Input: part model. Units: mm. Frame: model coordinates. Coordinates: 2 decimals unless noted, no trailing zeros. Write each loop counter-clockwise with the first axis right and the second up, starting at its lowest first coordinate (ties: lowest second). Pieces come first, ordered by that corner, then holes.
1) Section query B-B (z = 2.5). Output: boundary loops of the cut face in (x, y).
2) Section query D-D (x = -137). Output: boundary loops of the cut face in (y, z).
3) Section query C-C (y = 104). Output: boundary loops of the cut face in (x, z), then the cut area to 3 significant figures.
4) Section query A-A (x = -72.5). Output: boundary loops of the cut face in (y, z).
5) Line query: L1, parallel to Y at x = -47.5, z = 1.2; L2, parallel to X at y = 121, z = 0.85; L3, parallel to Y at x = -73, z = 1.75. Output: solid intervals per line, ascending.
from build123d import *

# Parameters (mm, degrees)
SKETCH_1_R      = 2.5
EXTRUDE_1_DEPTH = 4


with BuildPart() as part:
    # 草图1 → 凸台-拉伸1 (new body)
    with BuildSketch(Plane.XY):
        with BuildLine():
            Line((-11.50990482, 0), (-108.49009518, 0))
            ThreePointArc((-108.49009518, 0), (-117.621516615, 3.099699896), (-122.978982575, 11.117714323))
            Line((-122.978982575, 11.117714323), (-154.940506802, 130.399746626))
            ThreePointArc((-154.940506802, 130.399746626), (-152.351919512, 143.413453738), (-140.451619407, 149.282032303))
            Line((-140.451619407, 149.282032303), (20.451619407, 149.282032303))
            ThreePointArc((20.451619407, 149.282032303), (32.351919512, 143.413453738), (34.940506802, 130.399746626))
            Line((34.940506802, 130.399746626), (2.978982575, 11.117714323))
            ThreePointArc((2.978982575, 11.117714323), (-2.378483385, 3.099699896), (-11.50990482, 0))
        make_face()
        with Locations((-72.5, 81.282032303)):
            Circle(SKETCH_1_R, mode=Mode.SUBTRACT)
        with Locations((-72.5, 119.282032303)):
            Circle(SKETCH_1_R, mode=Mode.SUBTRACT)
        with Locations(Location((-47.5, 81.282032303, 0), (0, 0, 180))):
            Circle(SKETCH_1_R, mode=Mode.SUBTRACT)
        with Locations(Location((-47.5, 119.282032303, 0), (0, 0, 180))):
            Circle(SKETCH_1_R, mode=Mode.SUBTRACT)
    extrude(amount=EXTRUDE_1_DEPTH)


solid = part.part
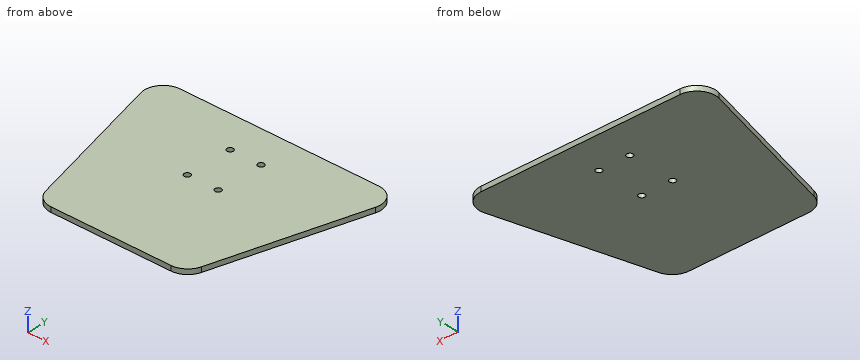
Answer:
1. outline: (-154.94, 130.4) - (-122.98, 11.12) arc R15 ccw to (-108.49, 0) - (-11.51, 0) arc R15 ccw to (2.98, 11.12) - (34.94, 130.4) arc R15 ccw to (20.45, 149.28) - (-140.45, 149.28) arc R15 ccw to start; hole circle Ø5 at (-72.5, 81.28); hole circle Ø5 at (-72.5, 119.28); hole circle Ø5 at (-47.5, 81.28); hole circle Ø5 at (-47.5, 119.28)
2. outline: (63.44, 0) - (149.28, 0) - (149.28, 4) - (63.44, 4) - close
3. outline: (-147.87, 0) - (27.87, 0) - (27.87, 4) - (-147.87, 4) - close
3. area: 703 mm2
4. outline: (0, 0) - (78.78, 0) - (78.78, 4) - (0, 4) - close; (83.78, 0) - (116.78, 0) - (116.78, 4) - (83.78, 4) - close; (121.78, 0) - (149.28, 0) - (149.28, 4) - (121.78, 4) - close
5. L1: y = 0 to 78.78, 83.78 to 116.78, 121.78 to 149.28
5. L2: x = -152.42 to -74.32, -70.68 to -49.32, -45.68 to 32.42
5. L3: y = 0 to 78.83, 83.73 to 116.83, 121.73 to 149.28
